from build123d import *

# Parameters (mm, degrees)
SKETCH_1_W               = 150
SKETCH_1_H               = 5
EXTRUDE_1_DEPTH          = 15
SKETCH_2_W               = 15
SKETCH_2_H               = 5
SKETCH_2_R               = 2.35
EXTRUDE_2_DEPTH          = 3
MIRROR_2_COPY_1_SKETCH_W = 15
MIRROR_2_COPY_1_SKETCH_H = 5
MIRROR_2_COPY_1_SKETCH_R = 2.35
MIRROR_2_COPY_1_DEPTH    = 3
SKETCH_3_W               = 16
SKETCH_3_H               = 20
CUT_EXTRUDE_1_DEPTH      = 53


with BuildPart() as part:
    # 草图1 → 凸台-拉伸1 (new body)
    with BuildSketch(Plane.XY):
        with Locations((75, 2.5)):
            Rectangle(SKETCH_1_W, SKETCH_1_H)
    extrude(amount=EXTRUDE_1_DEPTH)

    # 草图2 → 凸台-拉伸2 (add)
    # profile 1 of 4: a face of its own
    with BuildSketch(Plane.XY.offset(15)):
        with Locations((7.5, 2.5)):
            Rectangle(SKETCH_2_W, SKETCH_2_H)
    # profile 2 of 4: a face of its own
    with BuildSketch(Plane.XY.offset(15)):
        with BuildLine():
            Line((15, 0), (0, 0))
            Line((0, 0), (2.633939444, -11.149545417))
            ThreePointArc((2.633939444, -11.149545417), (6.921338951, -5.033597742), (12.5, -10))
            ThreePointArc((12.5, -10), (12.466402258, -10.578661049), (12.366060556, -11.149545417))
            Line((12.366060556, -11.149545417), (15, 0))
        make_face()
    # profile 3 of 4: a face of its own
    with BuildSketch(Plane.XY.offset(15)):
        with BuildLine():
            ThreePointArc((12.5, -10), (6.921338951, -5.033597742), (2.633939444, -11.149545417))
            ThreePointArc((2.633939444, -11.149545417), (7.5, -15), (12.366060556, -11.149545417))
            ThreePointArc((12.366060556, -11.149545417), (12.466402258, -10.578661049), (12.5, -10))
        make_face()
        with Locations((7.5, -10)):
            Circle(SKETCH_2_R, mode=Mode.SUBTRACT)
    # profile 4 of 4: a face of its own
    with BuildSketch(Plane.XY.offset(15)):
        with BuildLine():
            ThreePointArc((12.5, -10), (6.921338951, -5.033597742), (2.633939444, -11.149545417))
            ThreePointArc((2.633939444, -11.149545417), (7.5, -15), (12.366060556, -11.149545417))
            ThreePointArc((12.366060556, -11.149545417), (12.466402258, -10.578661049), (12.5, -10))
        make_face()
        with Locations((7.5, -10)):
            Circle(SKETCH_2_R, mode=Mode.SUBTRACT)
    extrude_2 = extrude(amount=EXTRUDE_2_DEPTH)

    # 镜向1: 凸台-拉伸2 across plane
    add(extrude_2.mirror(Plane(origin=(0, 0, 7.5), x_dir=(1, 0, 0), z_dir=(0, 0, -1))))

    # 镜向2: 凸台-拉伸2 across plane
    add(extrude_2.mirror(Plane.ZY.offset(-20)))

    # 镜向2 copy 1 sketch → 镜向2 copy 1 (add)
    # profile 1 of 4: a face of its own
    with BuildSketch(Plane(origin=(40, 0, 0), x_dir=(-1, 0, 0), z_dir=(0, 0, -1))):
        with Locations((7.5, 2.5)):
            Rectangle(MIRROR_2_COPY_1_SKETCH_W, MIRROR_2_COPY_1_SKETCH_H)
    # profile 2 of 4: a face of its own
    with BuildSketch(Plane(origin=(40, 0, 0), x_dir=(-1, 0, 0), z_dir=(0, 0, -1))):
        with BuildLine():
            Line((15, 0), (0, 0))
            Line((0, 0), (2.633939444, -11.149545417))
            ThreePointArc((2.633939444, -11.149545417), (6.921338951, -5.033597742), (12.5, -10))
            ThreePointArc((12.5, -10), (12.466402258, -10.578661049), (12.366060556, -11.149545417))
            Line((12.366060556, -11.149545417), (15, 0))
        make_face()
    # profile 3 of 4: a face of its own
    with BuildSketch(Plane(origin=(40, 0, 0), x_dir=(-1, 0, 0), z_dir=(0, 0, -1))):
        with BuildLine():
            ThreePointArc((12.5, -10), (6.921338951, -5.033597742), (2.633939444, -11.149545417))
            ThreePointArc((2.633939444, -11.149545417), (7.5, -15), (12.366060556, -11.149545417))
            ThreePointArc((12.366060556, -11.149545417), (12.466402258, -10.578661049), (12.5, -10))
        make_face()
        with Locations((7.5, -10)):
            Circle(MIRROR_2_COPY_1_SKETCH_R, mode=Mode.SUBTRACT)
    # profile 4 of 4: a face of its own
    with BuildSketch(Plane(origin=(40, 0, 0), x_dir=(-1, 0, 0), z_dir=(0, 0, -1))):
        with BuildLine():
            ThreePointArc((12.5, -10), (6.921338951, -5.033597742), (2.633939444, -11.149545417))
            ThreePointArc((2.633939444, -11.149545417), (7.5, -15), (12.366060556, -11.149545417))
            ThreePointArc((12.366060556, -11.149545417), (12.466402258, -10.578661049), (12.5, -10))
        make_face()
        with Locations((7.5, -10)):
            Circle(MIRROR_2_COPY_1_SKETCH_R, mode=Mode.SUBTRACT)
    extrude(amount=MIRROR_2_COPY_1_DEPTH)

    # 草图3 → 切除-拉伸1 (cut)
    with BuildSketch(Plane.ZY):
        with Locations((7.5, -10)):
            Rectangle(SKETCH_3_W, SKETCH_3_H)
    extrude(amount=-CUT_EXTRUDE_1_DEPTH, mode=Mode.SUBTRACT)


solid = part.part
Geometry: final body of the model. Coordinates: model frame, mm. A direction names the side the tool comes from. Give positions to 0.01 mm unless a question says otherwise; leave off trailing zeros. Order: outer loops, then holes, each group sorted by start corner. A loop starts at its lowest first (then second) coordinate and runs counter-clockwise, first axis right, second up. Notation, with made-up numbers: (-11.75, 61) -> (45.25, 61) arc R11 ccw to (45.25, 79) -> close; hole circle Ø8 at (7, 1). An arc over 180 degrees is marked (long way). Put each result on its own line as item: value.
Q1. Pin query (flat end, axial travel): pin 1 (1 mm diameter, centred on x = 35.5, z = -0.5, fed in from -Y); pin 2 (1 mm diameter, centred on y = -4, z = -0.5, fed in from -X); pin 3 (2.5 mm diameter, centred on x = 89, y = 2.5, fed in from -Z). Return the tip coordinate at first contact, or that it passes through.
Here are the results:
pin 1: stops at y = -14.33
pin 2: stops at x = 0.83
pin 3: stops at z = 0
Q2. Section B-B, the plane y = -6.25. Return loops of the section in (x, z), then the cut area to 3 significant figures.
Here are the results:
outline: (1.48, -3) -> (13.52, -3) -> (13.52, -0.5) -> (1.48, -0.5) -> close; (1.48, 15.5) -> (13.52, 15.5) -> (13.52, 18) -> (1.48, 18) -> close; (26.48, -3) -> (38.52, -3) -> (38.52, -0.5) -> (26.48, -0.5) -> close; (26.48, 15.5) -> (38.52, 15.5) -> (38.52, 18) -> (26.48, 18) -> close
area: 120 mm^2
Q3. Material intervals for L1, parallel to Y at x = 7.5, z = 16.3; L2, parallel to X at y = 0, z = 15.75; L3, parallel to Y at x = 17.5, z = 10, sorted ascending.
Here are the results:
L1: y = -15 to -12.35, -7.65 to 5
L2: x = 0 to 15, 25 to 40
L3: y = 0 to 5
Q4. Reachability of faces 1 (the face through (94, 3, 0)), 2 (the face through (13.665, -5.653, 16.732)), 3 (the face through (40, 2, 16)) from +Z, -Z, +X, -X, +Y, -Y: full face, straight path, thin tool, end or side. Return the list, or none.
Here are the results:
face 1: -Z, +X, +Y, -Y
face 2: +Z, -Z, -Y
face 3: +Z, +X, +Y, -Y
Q5. Section C-C, the plane x = 31.5. Return loops of the section in (y, z), then the cut area to 3 significant figures.
Here are the results:
outline: (-14.9, -3) -> (-12.13, -3) -> (-12.13, -0.5) -> (-14.9, -0.5) -> close; (-14.9, 15.5) -> (-12.13, 15.5) -> (-12.13, 18) -> (-14.9, 18) -> close; (-7.87, -3) -> (5, -3) -> (5, 18) -> (-7.87, 18) -> (-7.87, 15.5) -> (0, 15.5) -> (0, -0.5) -> (-7.87, -0.5) -> close
area: 158 mm^2
Q6. Draft query along X for faces 4 (the face through (40, 2, -1)), 5 (the face through (26.335, -5.653, -1.732)), 6 (the face through (7, -6, -0.5)). Return one class per face: released by +X, released by -X, zero draft, split by the parting line, or undercut.
Here are the results:
face 4: released by +X
face 5: undercut
face 6: zero draft
Q7. Section D-D, the plane z = 8.75. Return loops of the section in (x, y), then the cut area to 3 significant figures.
Here are the results:
outline: (0, 0) -> (150, 0) -> (150, 5) -> (0, 5) -> close
area: 750 mm^2
Q8. Section A-A, the plane x = 7.5. Return loops of the section in (y, z), then the cut area to 4 significant figures.
Here are the results:
outline: (-15, -3) -> (-12.35, -3) -> (-12.35, -0.5) -> (-15, -0.5) -> close; (-15, 15.5) -> (-12.35, 15.5) -> (-12.35, 18) -> (-15, 18) -> close; (-7.65, -3) -> (5, -3) -> (5, 18) -> (-7.65, 18) -> (-7.65, 15.5) -> (0, 15.5) -> (0, -0.5) -> (-7.65, -0.5) -> close
area: 156.5 mm^2
